For this review, use the dimensioned drawing (mm, ordinates from the lowest corner) and the shaded views. Give positions to 0.01 mm unless a question says otherwise; leave off trailing zeros. Write each loop counter-clockwise with the first axis right and the second up, starting at its lowest first coordinate (ties: lowest second). Pieces come first, ordered by that corner, then holes. Notation, with made-up numbers: (-23.75, 19.5) - (33.25, 19.5) arc R20 cw to (33.25, 54.5) - close; hole circle Ø7 at (40.25, 16). An arc over 180 degrees is marked (long way). One line per question, with ' | ' between items. Start each with the question number.
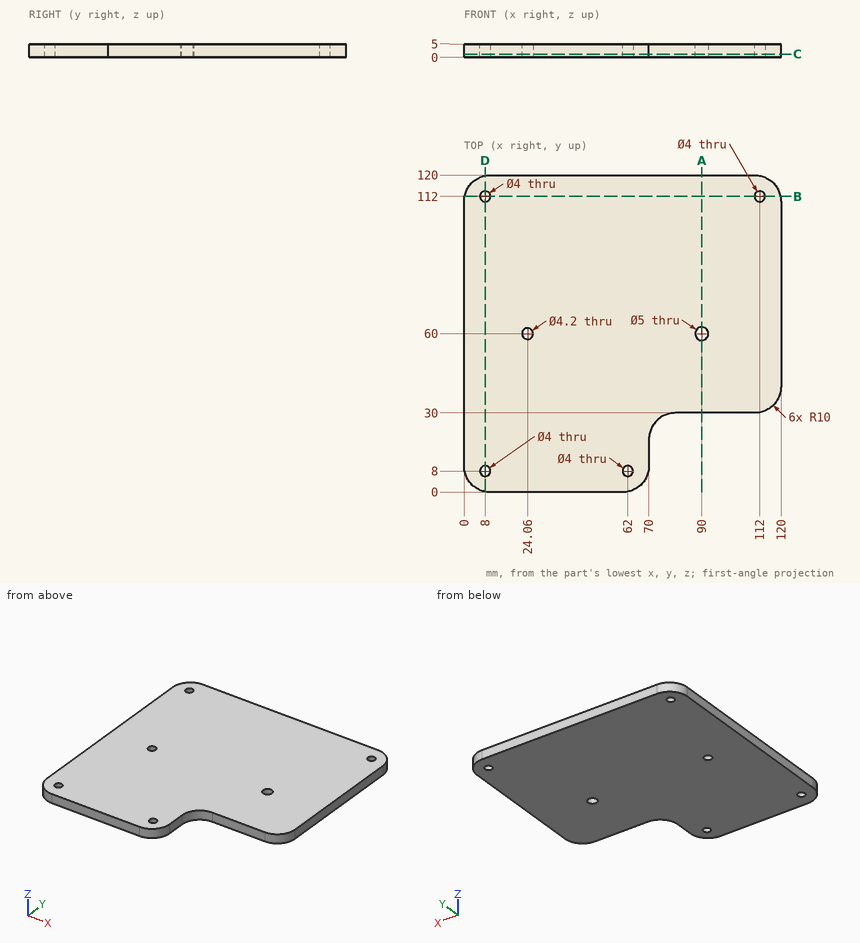
Item 1: Clearance check with flat-ended pins moving along their axes: P1, Ø3.5, axis at x = 62, y = 8, coming from the +Z side; P2, Ø1.5, axis at x = 89.5, z = 3.5, coming from the -Y side. State where each tip first meets the part, or that it passes through.
Item 2: Take a section at A-A (x = 90). Give the boundary of the cut face in (y, z).
Item 3: Take a section at B-B (y = 112). Give the boundary of the cut face in (x, z).
Item 4: Take a section at C-C (z = 1.15). Give the boundary of the cut face in (x, y), plus the area to 3 significant figures.
Item 5: For probe 1 along Y at (x, z) = (24.06, 1.1); probe 2 along Y at (x, z) = (90, 1); probe 3 along Y at (x, z) = (8, 1.2), list the stretches that pass through material, from the lowest coordinate up.
Check sheet entries:
1) P1: passes through | P2: stops at y = 30
2) outline: (30, 0) - (57.5, 0) - (57.5, 5) - (30, 5) - close; (62.5, 0) - (120, 0) - (120, 5) - (62.5, 5) - close
3) outline: (0.2, 0) - (6, 0) - (6, 5) - (0.2, 5) - close; (10, 0) - (110, 0) - (110, 5) - (10, 5) - close; (114, 0) - (119.8, 0) - (119.8, 5) - (114, 5) - close
4) outline: (0, 10) arc R10 ccw to (10, 0) - (60, 0) arc R10 ccw to (70, 10) - (70, 20) arc R10 cw to (80, 30) - (110, 30) arc R10 ccw to (120, 40) - (120, 110) arc R10 ccw to (110, 120) - (10, 120) arc R10 ccw to (0, 110) - close; hole circle Ø4 at (8, 8); hole circle Ø4 at (8, 112); hole circle Ø4.2 at (24.06, 60); hole circle Ø4 at (62, 8); hole circle Ø5 at (90, 60); hole circle Ø4 at (112, 112) | area: 12,700 mm^2
5) probe 1: y = 0 to 57.9, 62.1 to 120 | probe 2: y = 30 to 57.5, 62.5 to 120 | probe 3: y = 0.2 to 6, 10 to 110, 114 to 119.8
